The listing builds one solid part. Answer for the finished solid, in the listing's coordinates (mm). Face numbers are marked on the shaded views. A direction names the side the tool comes from. Round coordinates to 2 decimals unless told otherwise and drop trailing zeros. Order: outer loops, then holes, each group sorted by start corner. A loop starts at its lowest first (then second) coordinate and runs counter-clockwise, first axis right, second up. Notation, with made-up numbers: M 78.5,59.5 L 117.5,59.5 A24 cw 117.5,73.5 Z; hole C 67,9.25 d4. An arc over 180 degrees is marked long. Write item = value, one per line. Start each with the question number.
(1) Which of the six approach directions +Z, -Z, +X, -X, +Y, -Y give full straight-line access (tool end or side, diameter ignored) to the marked faces 1 and 2?
(2) A cutting plane is placed at A-A, the plane y = 135. Determine the outline of the cut face in (x, z), and give its area (3 significant figures).
(3) For a pull along Y with two mould halves and no side action, classify the marked faces 3, 4 and 5 as released by +Y, released by -Y, zero draft, split by the parting line, or undercut.
(4) A cutting plane is placed at C-C, the plane z = -21. Determine the outline of the cut face in (x, y), and give its area (3 significant figures).
(5) Straight lines are drawn through the part: probe 1 along Y at (x, z) = (-11, 10.5); probe 2 along Z at (x, y) = (0, 61); probe 3 along Y at (x, z) = (-13.5, -15). For each, find the intervals that lie inside material, in ascending order. Write a range as from..to.
(6) A cutting plane is placed at D-D, the plane y = 109.5. Determine the outline of the cut face in (x, z), and give its area (3 significant figures).
(7) A cutting plane is placed at B-B, the plane y = 43.5. Determine the outline of the cut face in (x, z).
(8) Each of these flat-tipped pins is pushed along its axis until it touches: pin 1 (7 mm diameter, centred on x = -9.5, y = 90, fed in from -Z); pin 2 (3 mm diameter, centred on x = -3, y = 113.5, fed in from -Z); pin 3 (4 mm diameter, centred on x = -7.66, z = -13.9, fed in from -Y); pin 4 (7.5 mm diameter, centred on x = 0, z = 0, fed in from +Y). Where does it stop, or does it pass through?
from build123d import *

# Parameters (mm, degrees)
F_1_4_20_TAPPED_HOLE1_D           = 5.1054
F_1_4_20_TAPPED_HOLE1_CSINK_D     = 7.62
F_1_4_20_TAPPED_HOLE1_CSINK_ANGLE = 100
BOSS_EXTRUDE1_DEPTH               = 88.9
SKETCH13_W                        = 6.096
SKETCH13_H                        = 30.48
BOSS_EXTRUDE2_DEPTH               = 55.88
CUT_EXTRUDE1_REACH                = 19.018
FILLET1_R                         = 7.62


with BuildPart() as part:
    # Sketch1 → Revolve1 (revolve)
    with BuildSketch(Plane.XY):
        Polygon((6.35, 19.05), (25.4, 19.05), (25.4, 25.4), (8.89, 25.4), (8.89, 114.3), (6.35, 114.3), align=None)
    revolve(axis=Axis((0, 131.17698584, 0), (0, -1, 0)))

    # 1/4-20 Tapped Hole1 (through all)
    with Locations(Plane(origin=(0, 25.4, 0), x_dir=(1, 0, 0), z_dir=(0, 1, 0))):
        with Locations((-8.212314406, -13.58578364), (-7.659476559, 13.904964719), (15.871790965, -0.319181079)):
            CounterSinkHole(F_1_4_20_TAPPED_HOLE1_D / 2, F_1_4_20_TAPPED_HOLE1_CSINK_D / 2, counter_sink_angle=F_1_4_20_TAPPED_HOLE1_CSINK_ANGLE)

    # Sketch12 → Boss-Extrude1 (add)
    with BuildSketch(Plane(origin=(0, 25.4, 0), x_dir=(1, 0, 0), z_dir=(0, 1, 0))):
        with BuildLine():
            Line((-5.480155107, -7), (-14.478, -7))
            Line((-14.478, -7), (-14.478, 7))
            Line((-14.478, 7), (-5.480155107, 7))
            ThreePointArc((-5.480155107, 7), (-8.89, 0), (-5.480155107, -7))
        make_face()
    extrude(amount=BOSS_EXTRUDE1_DEPTH)

    # Sketch13 → Boss-Extrude2 (add)
    with BuildSketch(Plane(origin=(0, 114.3, 0), x_dir=(1, 0, 0), z_dir=(0, 1, 0))):
        with Locations((-11.43, 0)):
            Rectangle(SKETCH13_W, SKETCH13_H)
    extrude(amount=BOSS_EXTRUDE2_DEPTH)

    # Sketch15 → Cut-Extrude1 (cut, up to next)
    with BuildSketch(Plane(origin=(-8.382, 0, 0), x_dir=(0, 0, -1), z_dir=(1, 0, 0)), mode=Mode.PRIVATE) as cut_extrude1_sk1:
        with BuildLine():
            Line((-11.132, 119.38), (-11.132, 165.1))
            ThreePointArc((-11.132, 165.1), (-9.1, 167.132), (-7.068, 165.1))
            Line((-7.068, 165.1), (-7.068, 119.38))
            ThreePointArc((-7.068, 119.38), (-9.1, 117.348), (-11.132, 119.38))
        make_face()
    cut_extrude1_tool1 = extrude(cut_extrude1_sk1.sketch, amount=-CUT_EXTRUDE1_REACH, mode=Mode.PRIVATE) & part.part
    add(cut_extrude1_tool1.solids().sort_by_distance((-8.382, 142.24, 9.1))[0], mode=Mode.SUBTRACT)
    # Sketch15 → Cut-Extrude1 (cut, up to next)
    with BuildSketch(Plane(origin=(-8.382, 0, 0), x_dir=(0, 0, -1), z_dir=(1, 0, 0)), mode=Mode.PRIVATE) as cut_extrude1_sk2:
        with BuildLine():
            Line((11.132, 119.38), (11.132, 165.1))
            ThreePointArc((11.132, 165.1), (9.1, 167.132), (7.068, 165.1))
            Line((7.068, 165.1), (7.068, 119.38))
            ThreePointArc((7.068, 119.38), (9.1, 117.348), (11.132, 119.38))
        make_face()
    cut_extrude1_tool2 = extrude(cut_extrude1_sk2.sketch, amount=-CUT_EXTRUDE1_REACH, mode=Mode.PRIVATE) & part.part
    add(cut_extrude1_tool2.solids().sort_by_distance((-8.382, 142.24, -9.1))[0], mode=Mode.SUBTRACT)

    # Fillet1
    fillet1_edges = [part.edges().sort_by_distance(p)[0] for p in [
        (-11.43, 114.3, 7),
        (-11.43, 114.3, -7),
    ]]
    fillet(fillet1_edges, radius=FILLET1_R)


solid = part.part
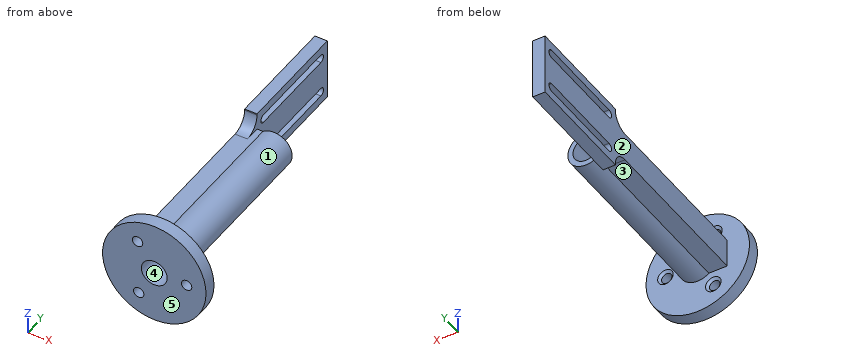
Reported:
q1.face_1 = +Y
q1.face_2 = +Z, -Z, -X, +Y
q2.outline = M -14.48,-15.24 L -8.38,-15.24 L -8.38,-11.13 L -14.48,-11.13 Z; M -14.48,-7.07 L -8.38,-7.07 L -8.38,7.07 L -14.48,7.07 Z; M -14.48,11.13 L -8.38,11.13 L -8.38,15.24 L -14.48,15.24 Z
q2.area = 136 mm²
q3.face_3 = undercut
q3.face_4 = zero draft
q3.face_5 = released by -Y
q4.outline = M -14.29,19.05 L 14.29,19.05 L 14.29,25.4 L -14.29,25.4 Z
q4.area = 181 mm²
q5.probe_1 = 19.05..25.4, 113.09..117.91, 166.57..170.18
q5.probe_2 = -8.89..-6.35, 6.35..8.89
q5.probe_3 = 19.05..25.4, 114.3..170.18
q6.outline = M -14.48,-7.54 L -8.38,-7.54 L -8.38,-7 L -5.48,-7 A8.89 ccw long -5.48,7 L -8.38,7 L -8.38,7.54 L -14.48,7.54 Z; hole C 0,0 d12.7
q6.area = 221 mm²
q7.outline = M -14.48,-7 L -5.48,-7 A8.89 ccw long -5.48,7 L -14.48,7 Z; hole C 0,0 d12.7
q8.pin_1 = -7
q8.pin_2 = -8.76
q8.pin_3 = 113.85
q8.pin_4 = through
